Can you work these out from the model? Positions are in its coordinate system, mm. A direction names the side the tool comes from. Coordinates: 2 decimals unless noted, no trailing zeros. Use a Markdown table: item, result. Add a question column.
(1) On a 3-axis mill with a long thin cutter (end or side, diameter ignored), from which of +Z, -Z, +X, -X, +Y, -Y can I reach the whole of each face in a straight line? I mean faces 1 (the flat face through (26.4, 20, 5)), 2 (the flat face through (3.6, 20, 5)), 3 (the conical face through (14.608, 28.236, 3.383)). Say none if no direction works.
(2) If I drill on L1, parallel to Y at x = 16, z = 3; L2, parallel to Y at x = 13.25, z = 2; L3, parallel to X at y = 32.5, z = 4.75, over which ranges is the centre line in solid material (lowest first)? Write a range as [from, to].
(3) For pin 1 Ø1.5 at (y, z) = (15, 5) entering from +X; pin 2 Ø1.5 at (x, y) = (15, 23.5) entering from +Z; pin 3 Ø5 at (x, y) = (10.5, 9.5) entering from -Z; pin 4 Ø3 at (x, y) = (1, 16) entering from +Z, each with a flat end and sliding along its axis, tell me the tip position at first contact or that it passes through.
(4) We'd pull the mould along X, two halves only. Please class faces 4 (the flat face through (0, 20, 2)), 5 (the flat face through (2, 20, 3.5)), 6 (the flat face through (16.2, 19.7, 5.6)): pulls with the +X half, pulls with the -X half, needs draft (parallel to the pull), parting line crosses it, or undercut.
```python
from build123d import *

# Parameters (mm, degrees)
F0_W     = 30
F0_H     = 40
F1_DEPTH = 7.1
F2_W     = 4
F2_H     = 25
F3_DEPTH = 1.5
F3_TAPER = 20
F4_W     = 3.6
F4_H     = 3.6
F5_DEPTH = 40.001
F6_R     = 1
F7_DEPTH = 20
F7_TAPER = -20


with BuildPart() as f1:
    # F0 (on Top) → F1 (new body)
    with BuildSketch(Plane.XY):
        with Locations((15, 20)):
            Rectangle(F0_W, F0_H)
    extrude(amount=F1_DEPTH)

    # F2 (on face) → F3 (cut)
    with BuildSketch(Plane.XY.offset(7.1)):
        with Locations((15, 20)):
            Rectangle(F2_W, F2_H)
    extrude(amount=-F3_DEPTH, taper=F3_TAPER, mode=Mode.SUBTRACT)

    # F4 (on face) → F5 (cut, through all)
    with BuildSketch(Plane.XZ):
        with Locations((1.8, 5.3)):
            Rectangle(F4_W, F4_H)
        Polygon((15, 7.1), (14.875, 7.1), (14.875, 6.8), (15, 6.8), (15.125, 6.8), (15.125, 7.1), align=None)
        with Locations((28.2, 5.3)):
            Rectangle(F4_W, F4_H)
    extrude(amount=-F5_DEPTH, mode=Mode.SUBTRACT)

    # F6 (on face) → F7 (cut)
    with BuildSketch(Plane.XY.offset(5.6)):
        with Locations((15, 30)):
            Circle(F6_R)
        with Locations((15, 20)):
            Circle(F6_R)
        with Locations((15, 10)):
            Circle(F6_R)
    extrude(amount=-F7_DEPTH, taper=F7_TAPER, mode=Mode.SUBTRACT)


solid = f1.part
```
Answers follow:
| question | item | result |
|---|---|---|
| 1 | face 1 | +Z, +X, +Y, -Y |
| 1 | face 2 | +Z, -X, +Y, -Y |
| 1 | face 3 | -Z |
| 2 | L1 | y = [0, 8.33], [11.67, 18.33], [21.67, 28.33], [31.67, 40] |
| 2 | L2 | y = [0, 8.49], [11.51, 18.49], [21.51, 28.49], [31.51, 40] |
| 2 | L3 | x = [3.6, 26.4] |
| 3 | pin 1 | stops at x = 26.4 |
| 3 | pin 2 | stops at z = 5.6 |
| 3 | pin 3 | stops at z = 0 |
| 3 | pin 4 | stops at z = 3.5 |
| 4 | face 4 | pulls with the -X half |
| 4 | face 5 | needs draft |
| 4 | face 6 | undercut |
